```python
from build123d import *

# Parameters (mm, degrees)
F2_DEPTH  = 38.1
F4_R      = 19.05
F5_DEPTH  = 38.101
F11_DEPTH = 117.475
F12_W     = 9.525
F12_H     = 6.35
F13_DEPTH = 6.35
F15_DEPTH = 12.7


# Not quite as in the source:
# - a feature of the source that left no trace in its solid (it failed there, or was rolled back) is left out


with BuildPart() as f2:
    # F1 (on Top) → F2 (new body)
    with BuildSketch(Plane.XY):
        with BuildLine():
            Line((-120.142, 381.762), (0, 381.762))
            Line((0, 381.762), (0, 444.5))
            Line((0, 444.5), (-30.734, 444.5))
            ThreePointArc((-30.734, 444.5), (-68.3812374672, 438.1220807393), (-101.8270568949, 419.700096432))
            ThreePointArc((-101.8270568949, 419.700096432), (-115.3236770577, 402.8258096141), (-120.142, 381.762))
        make_face()
        with BuildLine():
            Line((0, 444.5), (0, 381.762))
            Line((0, 381.762), (36.5448035283, 381.762))
            ThreePointArc((36.5448035283, 381.762), (32.2256329717, 389.9223670283), (30.734, 399.034))
            Line((30.734, 399.034), (30.734, 444.5))
            Line((30.734, 444.5), (0, 444.5))
        make_face()
        with BuildLine():
            Line((0, 381.762), (0, 295.402))
            Line((0, 295.402), (94.869, 295.402))
            ThreePointArc((94.869, 295.402), (96.466719449, 309.5567752573), (101.1794775617, 322.9992557201))
            Line((101.1794775617, 322.9992557201), (116.4239761752, 354.5902807248))
            ThreePointArc((116.4239761752, 354.5902807248), (120.430931673, 367.882227955), (120.142, 381.762))
            Line((120.142, 381.762), (91.175550227, 381.762))
            ThreePointArc((91.175550227, 381.762), (76.2148779155, 373.3684407202), (59.309, 370.459))
            ThreePointArc((59.309, 370.459), (46.6010649789, 373.440270055), (36.5448035283, 381.762))
            Line((36.5448035283, 381.762), (0, 381.762))
        make_face()
        with BuildLine():
            ThreePointArc((103.5459630182, 396.5232874828), (98.0699350262, 388.5483304334), (91.175550227, 381.762))
            Line((91.175550227, 381.762), (120.142, 381.762))
            ThreePointArc((120.142, 381.762), (118.0226976621, 389.4849479409), (114.552023257, 396.7022733785))
            ThreePointArc((114.552023257, 396.7022733785), (112.2345927331, 398.9686730826), (109.1004928586, 399.796))
            ThreePointArc((109.1004928586, 399.796), (105.8770068198, 398.9169814255), (103.5459630182, 396.5232874828))
        make_face()
        with BuildLine():
            Line((94.869, 295.402), (0, 295.402))
            Line((0, 295.402), (0, 0))
            Line((0, 0), (30.906359714, 0))
            ThreePointArc((30.906359714, 0), (123.5505287221, 38.3744712779), (161.925, 131.018640286))
            ThreePointArc((161.925, 131.018640286), (149.2199863218, 195.80132063), (112.9871937272, 250.9864434976))
            ThreePointArc((112.9871937272, 250.9864434976), (99.5727641582, 271.4175748279), (94.869, 295.402))
        make_face()
        with BuildLine():
            Line((0, 295.402), (-94.869, 295.402))
            ThreePointArc((-94.869, 295.402), (-99.5727641582, 271.4175748279), (-112.9871937272, 250.9864434976))
            ThreePointArc((-112.9871937272, 250.9864434976), (-149.2199863218, 195.80132063), (-161.925, 131.018640286))
            ThreePointArc((-161.925, 131.018640286), (-123.5505287221, 38.3744712779), (-30.906359714, 0))
            Line((-30.906359714, 0), (0, 0))
            Line((0, 0), (0, 295.402))
        make_face()
        with BuildLine():
            ThreePointArc((-104.887559724, 329.6362744337), (-97.4250853837, 313.2370573657), (-94.869, 295.402))
            Line((-94.869, 295.402), (0, 295.402))
            Line((0, 295.402), (0, 381.762))
            Line((0, 381.762), (-120.142, 381.762))
            ThreePointArc((-120.142, 381.762), (-116.2500581541, 354.6060190108), (-104.887559724, 329.6362744337))
        make_face()
    extrude(amount=F2_DEPTH)

    # F4 (on face) → F5 (cut, through all)
    with BuildSketch(Plane.XY.offset(38.1)):
        with Locations((-71.6915, 381.762)):
            Circle(F4_R)
        with BuildLine():
            Line((139.2962010965, 110.8024764079), (139.2962010965, 170.1017752607))
            ThreePointArc((139.2962010965, 170.1017752607), (129.7712010965, 186.5995592028), (110.7212010965, 186.5995592028))
            Line((110.7212010965, 186.5995592028), (66.675, 161.169473143))
            ThreePointArc((66.675, 161.169473143), (59.7022160579, 154.1966892009), (57.15, 144.6716892009))
            Line((57.15, 144.6716892009), (57.15, 108.5037669007))
            Line((57.15, 108.5037669007), (69.5417475728, 132.0304736397))
            ThreePointArc((69.5417475728, 132.0304736397), (65.9030700587, 154.5765309479), (88.5733379566, 151.8154392009))
            Line((88.5733379566, 151.8154392009), (107.8728631399, 162.9580252607))
            ThreePointArc((107.8728631399, 162.9580252607), (116.5483239896, 183.9024405039), (134.5337010965, 170.1017752607))
            ThreePointArc((134.5337010965, 170.1017752607), (130.3489892327, 159.9989871245), (120.2462010965, 155.8142752607))
            Line((120.2462010965, 155.8142752607), (120.2462010965, 125.0899764079))
            ThreePointArc((120.2462010965, 125.0899764079), (130.3489892327, 120.9052645441), (134.5337010965, 110.8024764079))
            ThreePointArc((134.5337010965, 110.8024764079), (125.4430565732, 97.4936316269), (109.7392514861, 101.1207066247))
            Line((109.7392514861, 101.1207066247), (90.3263274862, 83.23240717))
            ThreePointArc((90.3263274862, 83.23240717), (85.8817697832, 74.8654407377), (77.1799912803, 71.1185391723))
            Line((77.1799912803, 71.1185391723), (72.3922577123, 66.7068177967))
            ThreePointArc((72.3922577123, 66.7068177967), (79.2572186381, 66.5693077763), (85.725, 68.874606406))
            Line((85.725, 68.874606406), (129.7712010965, 94.3046924658))
            ThreePointArc((129.7712010965, 94.3046924658), (136.7439850386, 101.2774764079), (139.2962010965, 110.8024764079))
        make_face()
        with BuildLine():
            Line((69.5417475728, 132.0304736397), (57.15, 108.5037669007))
            Line((57.15, 108.5037669007), (57.15, 85.3723903481))
            ThreePointArc((57.15, 85.3723903481), (61.4446621425, 73.3232200567), (72.3922577123, 66.7068177967))
            Line((72.3922577123, 66.7068177967), (77.1799912803, 71.1185391723))
            ThreePointArc((77.1799912803, 71.1185391723), (85.8817697832, 74.8654407377), (90.3263274862, 83.23240717))
            Line((90.3263274862, 83.23240717), (109.7392514861, 101.1207066247))
            ThreePointArc((109.7392514861, 101.1207066247), (125.4430565732, 97.4936316269), (134.5337010965, 110.8024764079))
            ThreePointArc((134.5337010965, 110.8024764079), (130.3489892327, 120.9052645441), (120.2462010965, 125.0899764079))
            Line((120.2462010965, 125.0899764079), (120.2462010965, 155.8142752607))
            ThreePointArc((120.2462010965, 155.8142752607), (130.3489892327, 159.9989871245), (134.5337010965, 170.1017752607))
            ThreePointArc((134.5337010965, 170.1017752607), (116.5483239896, 183.9024405039), (107.8728631399, 162.9580252607))
            Line((107.8728631399, 162.9580252607), (88.5733379566, 151.8154392009))
            ThreePointArc((88.5733379566, 151.8154392009), (65.9030700587, 154.5765309479), (69.5417475728, 132.0304736397))
        make_face()
    extrude(amount=-F5_DEPTH, mode=Mode.SUBTRACT)

    # F10 (on face) → F11 (cut)
    with BuildSketch(Plane(origin=(0, 441.123523107, -38.5933074865), x_dir=(-1, 0, 0), z_dir=(0, 0.9961946981, -0.0871557427))):
        with BuildLine():
            Line((19.05, 76.6957456486), (-19.05, 76.6957456486))
            Line((-19.05, 76.6957456486), (-19.05, 67.1707456486))
            ThreePointArc((-19.05, 67.1707456486), (-15.3302561211, 58.1904895276), (-6.35, 54.4707456486))
            Line((-6.35, 54.4707456486), (0, 54.4707456486))
            Line((0, 54.4707456486), (6.35, 54.4707456486))
            ThreePointArc((6.35, 54.4707456486), (15.3302561211, 58.1904895276), (19.05, 67.1707456486))
            Line((19.05, 67.1707456486), (19.05, 76.6957456486))
        make_face()
    extrude(amount=-F11_DEPTH, mode=Mode.SUBTRACT)

    # F12 (on face) → F13 (cut)
    with BuildSketch(Plane.XY.offset(38.1)):
        Polygon((-34.29, 299.5168), (0, 299.5168), (0, 317.8302), (-34.29, 317.8302), (-34.29, 311.4802), (-34.29, 308.3052), align=None)
        Polygon((0, 317.8302), (0, 299.5168), (34.29, 299.5168), (34.29, 311.4802), (34.29, 317.8302), align=None)
        Polygon((0, 229.6668), (-34.29, 229.6668), (-34.29, 217.7034), (-34.29, 211.3534), (0, 211.3534), align=None)
        Polygon((34.29, 229.6668), (0, 229.6668), (0, 211.3534), (34.29, 211.3534), (34.29, 217.7034), align=None)
        with Locations((-39.0525, 214.5284)):
            Rectangle(F12_W, F12_H)
        Polygon((34.29, 211.3534), (0, 211.3534), (0, 193.04), (34.29, 193.04), (34.29, 205.0034), align=None)
        Polygon((0, 193.04), (0, 211.3534), (-34.29, 211.3534), (-34.29, 205.0034), (-34.29, 193.04), align=None)
        with Locations((-39.0525, 208.1784)):
            Rectangle(F12_W, F12_H)
        with Locations((39.0525, 214.5284)):
            Rectangle(F12_W, F12_H)
        Polygon((0, 336.1436), (0, 317.8302), (34.29, 317.8302), (34.29, 324.1802), (34.29, 336.1436), align=None)
        Polygon((-34.29, 317.8302), (0, 317.8302), (0, 336.1436), (-34.29, 336.1436), (-34.29, 324.1802), align=None)
        with Locations((39.0525, 208.1784)):
            Rectangle(F12_W, F12_H)
        Polygon((-43.815, 308.3052), (-34.29, 308.3052), (-34.29, 311.4802), (-34.29, 317.8302), (-43.815, 317.8302), (-43.815, 311.4802), align=None)
        with Locations((39.0525, 314.6552)):
            Rectangle(F12_W, F12_H)
        with Locations((39.0525, 321.0052)):
            Rectangle(F12_W, F12_H)
        with Locations((-39.0525, 321.0052)):
            Rectangle(F12_W, F12_H)
    extrude(amount=-F13_DEPTH, mode=Mode.SUBTRACT)

    # F14 (on face) → F15 (cut)
    with BuildSketch(Plane.XY.offset(38.1)):
        with BuildLine():
            Line((-54.0675192427, 388.9937219434), (-58.0760770823, 368.4382333114))
            Line((-58.0760770823, 368.4382333114), (57.15, 135.255))
            Line((57.15, 135.255), (57.15, 144.6716892009))
            ThreePointArc((57.15, 144.6716892009), (58.1362792436, 150.7218538627), (60.9929913317, 156.1455458918))
            Line((60.9929913317, 156.1455458918), (-54.0675192427, 388.9937219434))
        make_face()
    extrude(amount=-F15_DEPTH, mode=Mode.SUBTRACT)


solid = f2.part
```
CAD build for the part. Positions are in the model's coordinates, mm. A direction names the side the tool comes from. Coordinates: 2 decimals unless noted, no trailing zeros. Order: outer loops, then holes, each group sorted by start corner. A loop starts at its lowest first (then second) coordinate and runs counter-clockwise, first axis right, second up.
(1) Mould opens along Y. For faces 1 (the face through (122.526, 37.361, 18.783)), 2 (the face through (-67.87, 438.3, 18.78)), 3 (the face through (136.7, 101.2, 19.3)) say: released by +Y, released by -Y, zero draft, split by the parting line, or undercut.
Solution:
face 1: released by -Y
face 2: released by +Y
face 3: undercut
(2) Which spindle directions (+Z, -Z, +X, -X, +Y, -Y) get a long thin tool onto all of the face, cutting with end or side? Do faces 4 (the face through (57.15, 115, 19)), 5 (the face through (108.695, 338.574, 18.783)), 6 (the face through (-15.231, 387.797, 24.386)), 7 (the face through (-116.36, 354.98, 18.78)). Say none if no direction does.
Solution:
face 4: +Z, -Z
face 5: +Z, -Z, +X
face 6: +Z, +Y
face 7: +Z, -Z, -X
(3) Saw through at D-D, the plane y = 245.5. Write the cut outline in (x, z).
Solution:
outline: (-118.13, 0) - (118.13, 0) - (118.13, 38.1) - (16.84, 38.1) - (16.84, 25.4) - (2.67, 25.4) - (2.67, 38.1) - (-118.13, 38.1) - close
(4) Saw through at C-C, the plane x = -71. Write the cut outline in (y, z).
Solution:
outline: (6.29, 0) - (362.72, 0) - (362.72, 38.1) - (6.29, 38.1) - close; (400.8, 0) - (437.17, 0) - (437.17, 38.1) - (400.8, 38.1) - close
(5) Saw through at B-B, the plane y = 106. Write the cut outline in (x, z), and give its area (3 significant figures).
Solution:
outline: (-159.51, 0) - (57.15, 0) - (57.15, 38.1) - (-159.51, 38.1) - close; (138.68, 0) - (159.51, 0) - (159.51, 38.1) - (138.68, 38.1) - close
area: 9,050 mm2
(6) Saw through at A-A, the plane z = 11. Count the separate pieces of the cut face and the enclosed holes in it, and give its area (3 significant figures).
Solution:
separate pieces: 1
enclosed holes: 2
area: 97,000 mm2
(7) Pin check, flat tips, straight feed: pin 1 Ø3 at (y, z) = (211.5, 33.5) entering from +X; pin 2 Ø16 at (x, y) = (-33.5, 316) entering from +Z; pin 3 Ø1 at (y, z) = (91, 16) entering from +X; pin 4 Ø7 at (x, z) = (-38, 36.5) entering from +Y. Stop position of each tip, or through.
Solution:
pin 1: stops at x = 142.66
pin 2: stops at z = 38.1
pin 3: stops at x = 155.82
pin 4: stops at y = 444.44
(8) Drill centre lines: L1, parallel to X at y = 379.5, z = 19; L2, parallel to X at y = 391, z = 33.5; L3, parallel to Z at x = 40, y = 206. Where is each one in solid material? Low to high.
Solution:
L1: x = -120.12 to -90.61, -52.78 to 38.45, 88.17 to 120.49
L2: x = -119.25 to -88.35, -55.03 to -19.05, 19.05 to 31.89, 100 to 117.42
L3: z = 0 to 31.75
